Part model, mm, in its own coordinate system. Face numbers are marked on the shaded views. A direction names the side the tool comes from. Give positions to 0.01 mm unless a question says otherwise; leave off trailing zeros. Write each loop counter-clockwise with the first axis right and the second up, starting at its lowest first coordinate (ties: lowest second). Pieces come first, ordered by that corner, then holes. Notation, with made-up numbers: M 38.25,-33 L 81.25,-33 A9 cw 81.25,-29 Z; hole C 10,16 d2. An arc over 180 degrees is marked long. Write item = value, one per line. Start each with the question number.
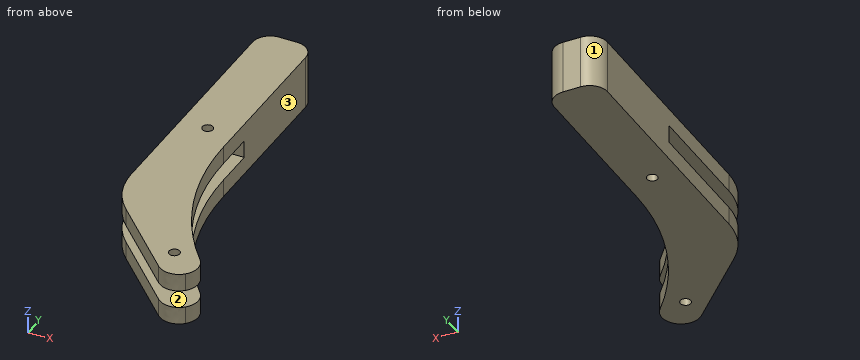
from build123d import *

# Parameters (mm, degrees)
BOSS_EXTRU_1_DEPTH      = 15
CONG_1_R                = 72
CONG_2_R                = 20
ESQUISSE2_W             = 5
ESQUISSE2_H             = 70
ENL_V_MAT_EXTRU_1_DEPTH = 90.086452972
ESQUISSE3_R             = 1.5
ENL_V_MAT_EXTRU_2_DEPTH = 90.086452972
CONG_3_R                = 5
CONG_4_START            = 9
CONG_4_DEPTH            = 7
CONG_5_START            = -1
CONG_5_DEPTH            = 7


with BuildPart() as part:
    # Esquisse1 → Boss.-Extru.1 (new body)
    with BuildSketch(Plane.XY):
        Polygon((0, 0), (0, 80), (15, 80), (15, 0), (36.213203436, -21.213203436), (28.713203436, -28.713203436), align=None)
    extrude(amount=BOSS_EXTRU_1_DEPTH)

    # Congé1
    cong_1_edges = [part.edges().sort_by_distance(p)[0] for p in [
        (15, 0, 7.5),
    ]]
    fillet(cong_1_edges, radius=CONG_1_R)

    # Congé2
    cong_2_edges = [part.edges().sort_by_distance(p)[0] for p in [
        (0, 0, 7.5),
    ]]
    fillet(cong_2_edges, radius=CONG_2_R)

    # Esquisse2 → Enlèv. mat.-Extru.1 (cut, through all)
    with BuildSketch(Plane(origin=(0, 0, 0), x_dir=(0, 0, -1), z_dir=(1, 0, 0))):
        with Locations((-7.5, 6.286796564)):
            Rectangle(ESQUISSE2_W, ESQUISSE2_H)
    extrude(amount=ENL_V_MAT_EXTRU_1_DEPTH, mode=Mode.SUBTRACT)

    # Esquisse3 → Enlèv. mat.-Extru.2 (cut, through all)
    with BuildSketch(Plane.XY.offset(15)):
        with Locations((7.61728785, 35.6306026)):
            Circle(ESQUISSE3_R)
        with Locations((25.630175336, -17.654095912)):
            Circle(ESQUISSE3_R)
    extrude(amount=-ENL_V_MAT_EXTRU_2_DEPTH, mode=Mode.SUBTRACT)

    # Congé3
    cong_3_edges = [part.edges().sort_by_distance(p)[0] for p in [
        (0, 80, 7.5),
        (15, 80, 7.5),
    ]]
    fillet(cong_3_edges, radius=CONG_3_R)

    # Congé4: read off the stored shape, not the designer's step
    # Congé4 outline → Congé4 (cut)
    with BuildSketch(Plane.XY.offset(CONG_4_START)):
        with BuildLine():
            ThreePointArc((36.088311756, -21.088311756), (34.40105692, -19.343189251), (32.773587535, -17.542182633))
            add(Edge.make_bspline(
                [(32.773587535, -17.542182633), (34.472065544, -19.486683464), (34.913542675, -22.512864199), (32.525386467, -24.901020408)],
                knots=[0, 0, 0, 0, 0.49128121, 0.49128121, 0.49128121, 0.49128121], degree=3, weights=[1, 0.683519634, 0.522520126, 0.517001474]))
            Line((32.525386467, -24.901020408), (36.213203437, -21.213203437))
            Line((36.213203437, -21.213203437), (36.088311756, -21.088311756))
        make_face()
        with BuildLine():
            Line((28.713203437, -28.713203437), (32.525386467, -24.901020408))
            add(Edge.make_bspline(
                [(32.525386467, -24.901020408), (29.99813373, -27.428273144), (26.823045344, -26.823045346), (24.901020406, -24.901020406)],
                knots=[0.49128121, 0.49128121, 0.49128121, 0.49128121, 1, 1, 1, 1], degree=3, weights=[0.517001474, 0.511286943, 0.672286452, 1]))
            Line((24.901020406, -24.901020406), (28.713203437, -28.713203437))
        make_face()
    extrude(amount=CONG_4_DEPTH, mode=Mode.SUBTRACT)

    # Congé5: read off the stored shape, not the designer's step
    # Congé5 outline → Congé5 (cut)
    with BuildSketch(Plane.XY.offset(CONG_5_START)):
        with BuildLine():
            ThreePointArc((36.088311755, -21.088311755), (34.401056918, -19.343189249), (32.773587531, -17.542182629))
            add(Edge.make_bspline(
                [(32.773587531, -17.542182629), (34.472065541, -19.486683459), (34.913542673, -22.512864192), (32.525386468, -24.901020401)],
                knots=[0, 0, 0, 0, 0.49128121, 0.49128121, 0.49128121, 0.49128121], degree=3, weights=[1, 0.683519634, 0.522520126, 0.517001474]))
            Line((32.525386468, -24.901020401), (36.213203436, -21.213203436))
            Line((36.213203436, -21.213203436), (36.088311755, -21.088311755))
        make_face()
        with BuildLine():
            Line((28.713203436, -28.713203436), (32.525386468, -24.901020401))
            add(Edge.make_bspline(
                [(32.525386468, -24.901020401), (29.998133731, -27.428273143), (26.823045342, -26.823045344), (24.901020402, -24.901020402)],
                knots=[0.49128121, 0.49128121, 0.49128121, 0.49128121, 1, 1, 1, 1], degree=3, weights=[0.517001474, 0.511286943, 0.672286451, 1]))
            Line((24.901020402, -24.901020402), (28.713203436, -28.713203436))
        make_face()
    extrude(amount=CONG_5_DEPTH, mode=Mode.SUBTRACT)


solid = part.part
Q1. Slice it at B-B (z = 8). Give the cut face in (x, y), and give its area (3 significant figures).
Q2. Probe line 1 along Z through (x, y) = (9.5, 32); line 2 along Y through (x, z) = (7, 7.75); line 3 along X through (y, z) = (-19, 3.75). List the from-to ranges inside material, lowest first.
Q3. Drop flat-ended pins along their axis: P1, Ø1.8, axis at x = 25.63, y = -17.65, coming from the -Z side; P2, Ø6, axis at x = 15, z = 9.5, coming from the -Y side; P3, Ø2.5, axis at x = 10.5, z = 8, coming from the -Y side; P4, Ø1, axis at x = 25.5, z = 4.5, coming from the -Y side. Give the stop position or say it passes through.
Q4. Slice it at D-D (y = -4). Give the cut face in (x, z), and give its area (3 significant figures).
Q5. Slice it at C-C (x = 11.5). Give the cut face in (y, z).
Q6. Tool access for the marked faces 1, 2 and 3: list every direction of +Z, -Z, +X, -X, +Y, -Y with a clear straight run to the whole face (end or side of a thin tool).
Q7. Slice it at A-A (y = -15). Give the cut face in (x, z), and give its area (3 significant figures).
Working result:
q1.outline = M 0,41.29 L 15,41.29 L 15,75 A5 ccw 10,80 L 5,80 A5 ccw 0,75 Z
q1.area = 570 mm2
q2.line_1 = 0 to 5, 10 to 15
q2.line_2 = 41.29 to 80
q2.line_3 = 19 to 24.97, 26.29 to 33.68
q3.P1 = through
q3.P2 = -17.96
q3.P3 = 41.29
q3.P4 = -25.75
q4.outline = M 4.22,0 L 23.44,0 L 23.44,5 L 4.22,5 Z; M 4.22,10 L 23.44,10 L 23.44,15 L 4.22,15 Z
q4.area = 192 mm2
q5.outline = M -11.5,0 L 79.77,0 L 79.77,15 L -11.5,15 L -11.5,10 L 41.29,10 L 41.29,5 L -11.5,5 Z
q6.face_1 = +Z, -Z, -X, +Y
q6.face_2 = +X, -X, -Y
q6.face_3 = +Z, -Z, +X, +Y
q7.outline = M 15,0 L 30.65,0 L 30.65,5 L 15,5 Z; M 15,10 L 30.65,10 L 30.65,15 L 15,15 Z
q7.area = 157 mm2
